```python
from build123d import *

# Parameters (mm, degrees)
SKETCH1_R           = 23
SKETCH1_R_2         = 1.75
BOSS_EXTRUDE1_DEPTH = 9.5
SKETCH1_3_R         = 25.5
SKETCH1_3_R_2       = 23
BOSS_EXTRUDE2_DEPTH = 1
SKETCH1_4_R         = 12.5
CUT_EXTRUDE1_DEPTH  = 5


with BuildPart() as part:
    # Sketch1 → Boss-Extrude1 (new body)
    with BuildSketch(Plane.XY):
        Circle(SKETCH1_R)
        with Locations((0, 8)):
            Circle(SKETCH1_R_2, mode=Mode.SUBTRACT)
        with Locations((8, 0)):
            Circle(SKETCH1_R_2, mode=Mode.SUBTRACT)
        with Locations((0, -8)):
            Circle(SKETCH1_R_2, mode=Mode.SUBTRACT)
        with Locations((-8, 0)):
            Circle(SKETCH1_R_2, mode=Mode.SUBTRACT)
    extrude(amount=BOSS_EXTRUDE1_DEPTH)

    # Sketch1_3 → Boss-Extrude2 (add)
    with BuildSketch(Plane.XY):
        Circle(SKETCH1_3_R)
        Circle(SKETCH1_3_R_2, mode=Mode.SUBTRACT)
    extrude(amount=BOSS_EXTRUDE2_DEPTH)

    # Sketch1_4 → Cut-Extrude1 (cut)
    with BuildSketch(Plane.XY):
        Circle(SKETCH1_4_R)
    extrude(amount=CUT_EXTRUDE1_DEPTH, mode=Mode.SUBTRACT)


solid = part.part
```
Input: part model. Units: mm. Frame: model coordinates. A direction names the side the tool comes from. Round coordinates to 2 decimals unless told otherwise and drop trailing zeros. Order: outer loops, then holes, each group sorted by start corner. A loop starts at its lowest first (then second) coordinate and runs counter-clockwise, first axis right, second up. Notation, with made-up numbers: (89.5, 31.25) - (132.5, 31.25) arc R19 cw to (132.5, 60.25) - close; hole circle Ø7 at (83.25, -27). An arc over 180 degrees is marked (long way). Answer in a Markdown table with one row per item.
Item 1: Section query C-C (z = 8.75). Return the cut outline in (x, y).
Model answer:
| item | result |
|---|---|
| outline | circle Ø46 at (0, 0); hole circle Ø3.5 at (-8, 0); hole circle Ø3.5 at (0, -8); hole circle Ø3.5 at (0, 8); hole circle Ø3.5 at (8, 0) |
Item 2: Reachability of faces 4 (the cylindrical face through (-2.994, 22.804, 5.19)), 5 (the cylindrical face through (-0.228, 9.735, 7.219)), 6 (the flat face through (0, 0, 5)) from +Z, -Z, +X, -X, +Y, -Y: full face, straight path, thin tool, end or side. Return the list, or none.
Model answer:
| item | result |
|---|---|
| face 4 | +Z |
| face 5 | +Z, -Z |
| face 6 | -Z |
Item 3: Mould query, pull axis Z, two halves, no side actions, for faces 1 (the flat face through (0, 0, 9.5)), 2 (the cylindrical face through (9.669, 0.526, 7.219)), 3 (the flat face through (5, 12, 0)). Classes: released by +Z, released by -Z, zero draft, split by the parting line, or undercut.
Model answer:
| item | result |
|---|---|
| face 1 | released by +Z |
| face 2 | zero draft |
| face 3 | released by -Z |
Item 4: Section query D-D (x = 8). Return the cut outline in (y, z), then the cut area to 3 significant figures.
Model answer:
| item | result |
|---|---|
| outline | (-24.21, 0) - (-9.6, 0) - (-9.6, 5) - (-1.75, 5) - (-1.75, 9.5) - (-21.56, 9.5) - (-21.56, 1) - (-24.21, 1) - close; (1.75, 5) - (9.6, 5) - (9.6, 0) - (24.21, 0) - (24.21, 1) - (21.56, 1) - (21.56, 9.5) - (1.75, 9.5) - close |
| area | 303 mm² |
Item 5: Section query A-A (x = 0). Return the cut outline in (y, z), then the cut area to 4 significant figures.
Model answer:
| item | result |
|---|---|
| outline | (-25.5, 0) - (-12.5, 0) - (-12.5, 5) - (-9.75, 5) - (-9.75, 9.5) - (-23, 9.5) - (-23, 1) - (-25.5, 1) - close; (-6.25, 5) - (6.25, 5) - (6.25, 9.5) - (-6.25, 9.5) - close; (9.75, 5) - (12.5, 5) - (12.5, 0) - (25.5, 0) - (25.5, 1) - (23, 1) - (23, 9.5) - (9.75, 9.5) - close |
| area | 285.5 mm² |
Item 6: Line query: line 1 (Y direction, x = 0, z = 8.35); line 2 (Y direction, x = 0, z = 1.55); line 3 (Z direction, x = 6.5, y = 23.5). Output: solid intervals per line, ascending.
Model answer:
| item | result |
|---|---|
| line 1 | y = -23 to -9.75, -6.25 to 6.25, 9.75 to 23 |
| line 2 | y = -23 to -12.5, 12.5 to 23 |
| line 3 | z = 0 to 1 |
Item 7: Pin query (flat end, axial travel): pin 1 (4.5 mm diameter, centred on x = 0, y = -8, fed in from -Z); pin 2 (3 mm diameter, centred on x = -8, y = 0, fed in from +Z); pin 3 (1 mm diameter, centred on y = 3, z = 5.5, fed in from +X); pin 4 (3 mm diameter, centred on y = -17, z = 3, fed in from +X). Return the tip coordinate at first contact, or that it passes through.
Model answer:
| item | result |
|---|---|
| pin 1 | stops at z = 5 |
| pin 2 | passes through |
| pin 3 | stops at x = 22.86 |
| pin 4 | stops at x = 16.99 |
